For this review, take the finished solid that the model builds, in its own axes (mm). Coordinates: 2 decimals unless noted, no trailing zeros. Loops run counter-clockwise (first coordinate to the right, second up) from the corner with the lowest first, then second, coordinate; pieces in that order, holes last. Notation, with made-up numbers: M -3.5,65.25 L 47.5,65.25 A29 ccw 47.5,93.25 Z; hole C -9,-9 d11. An arc over 180 degrees is marked long. Write item = value, one per line.
Autodesk Inventor part; units mm, degrees
ref_plane "YZ Plane" through (0, 0, 0) normal (1, 0, 0) x (0, 1, 0)
ref_plane "XZ Plane" through (0, 0, 0) normal (0, 1, 0) x (-1, 0, 0)
ref_plane "XY Plane" through (0, 0, 0) normal (0, 0, 1) x (1, 0, 0)
sketch "Szkic1" plane through (0, 0, 0) normal (0, 1, 0) x (-1, 0, 0)
  line L0 (-159, -101.5) -> (159, -101.5)
  line L1 (159, -101.5) -> (159, 101.5)
  line L2 (159, 101.5) -> (-159, 101.5)
  line L3 (-159, 101.5) -> (-159, -101.5)
  line L4 (-159, -101.5) -> (159, 101.5) construction
  line L5 (159, -101.5) -> (-159, 101.5) construction
  circle A0 centre (0, 66.5) radius 10.5
  point P0 (0, 0)
  dimension "d0" = 318
  dimension "d1" = 203
  dimension "d2" = 21
  dimension "d3" = 35
  dimension "d4" = 159
extrude "Wyciągnięcie proste1" add sketch "Szkic1" along normal mid plane 3
properties part number "scina_prawa"
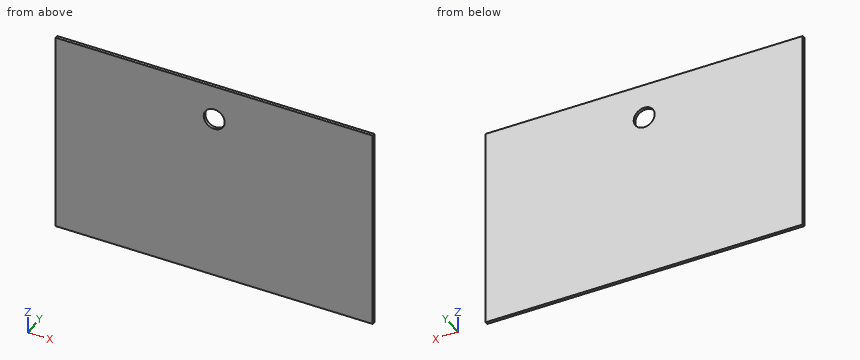
Q1. For pin 1 Ø12.5 at (x, z) = (0, 66.5) entering from +Y, flat-tipped, find the tip position at first contact; note if it passes through.
Solved:
pin_1 = through
Q2. Add section A-A (z = 66.5). Write out the cut boundary in (x, y), and give its area (3 significant figures).
Solved:
outline = M -159,-1.5 L -10.5,-1.5 L -10.5,1.5 L -159,1.5 Z; M 10.5,-1.5 L 159,-1.5 L 159,1.5 L 10.5,1.5 Z
area = 891 mm²
Q3. Add section B-B (x = 0). Write out the cut boundary in (y, z), and give its area (3 significant figures).
Solved:
outline = M -1.5,-101.5 L 1.5,-101.5 L 1.5,56 L -1.5,56 Z; M -1.5,77 L 1.5,77 L 1.5,101.5 L -1.5,101.5 Z
area = 546 mm²
Q4. For line 1 along Z through (x, y) = (0, 0.8); line 2 along Z through (x, y) = (6, 0.4); line 3 along X through (y, z) = (1.3, 69), list the stretches that pass through material, from the lowest coordinate up.
Solved:
line_1 = -101.5 to 56, 77 to 101.5
line_2 = -101.5 to 57.88, 75.12 to 101.5
line_3 = -159 to -10.2, 10.2 to 159
